Read the model definition and answer for the solid it produces. Units are mm, in the model's axes. Coordinates: 2 decimals unless noted, no trailing zeros. Write each loop counter-clockwise with the first axis right and the second up, starting at its lowest first coordinate (ties: lowest second). Pieces come first, ordered by that corner, then holes.
Item 1: Section B-B (z = 0) is taken. Give the vertices of the cut face in (x, y), then the cut area to 3 significant figures.
Item 2: Section D-D (y = 9) is taken. Give the vertices of the cut face in (x, z).
Item 3: Section C-C (y = 0) is taken. Give the vertices of the cut face in (x, z).
Item 4: Section A-A (x = 0) is taken. Give the vertices of the cut face in (y, z).
Item 5: Each of these flat-tipped pins is pushed along its axis until it touches: P1, Ø5, axis at y = -30, z = -0.5, coming from the -X side; P2, Ø5, axis at x = -25, y = -25.5, coming from the +Z side; P3, Ø3, axis at y = -15.5, z = 20.5, coming from the -X side. Where does it stop, or does it pass through?
Item 6: Determine the mould class of faces 1 (the face through (1, 40, -1)), 2 (the face through (1, -40, -1)), 3 (the face through (13.41, 32.33, 0.55)) for opening direction Y: released by +Y, released by -Y, zero draft, split by the parting line, or undercut.
Item 7: Straight lines are drawn through the part: probe 1 along Y at (x, z) = (0, -4); probe 2 along X at (y, z) = (0, -1); probe 3 along X at (y, z) = (0, -14.5). For each, find the intervals that lie inside material, in ascending order.
from build123d import *

# Parameters (mm, degrees)
SCHIZZO1_R        = 39
ESTRUSIONE1_DEPTH = 40
SCHIZZO3_R        = 35
ESTRUSIONE3_DEPTH = 40
SMUSSO1_SIZE      = 1


with BuildPart() as part:
    # Schizzo1 → Estrusione1 (new, symmetric)
    with BuildSketch(Plane(origin=(0, 0, 0), x_dir=(1, 0, 0), z_dir=(0, 1, 0))):
        with Locations(Location((0, 0, 0), (0, 0, 270))):
            Circle(SCHIZZO1_R)
    extrude(amount=ESTRUSIONE1_DEPTH, both=True)

    # Schizzo3 → Estrusione3 (cut, symmetric)
    with BuildSketch(Plane.XY):
        with Locations(Location((0, 0, 0), (0, 0, 90))):
            Circle(SCHIZZO3_R)
    extrude(amount=ESTRUSIONE3_DEPTH, both=True, mode=Mode.SUBTRACT)

    # Smusso1
    smusso1_edges = [part.edges().sort_by_distance(p)[0] for p in [
        (0, 40, -39),
    ]]
    chamfer(smusso1_edges, length=SMUSSO1_SIZE)


solid = part.part
Established:
1. outline: (-39, -40) - (39, -40) - (39, 39) - (38, 40) - (-38, 40) - (-39, 39) - close; hole circle Ø70 at (0, 0)
1. area: 2,390 mm2
2. outline: (-33.82, -19.42) - (-33.82, 19.42) arc R39 ccw to start; (33.82, -19.42) arc R39 ccw to (33.82, 19.42) - close
3. outline: (-35, -17.2) - (-35, 17.2) arc R39 ccw to start; (35, -17.2) arc R39 ccw to (35, 17.2) - close
4. outline: (-40, -39) - (-35, -39) - (-35, 39) - (-40, 39) - close; (35, -39) - (39, -39) - (40, -38) - (40, 38) - (39, 39) - (35, 39) - close
5. P1: stops at x = -39
5. P2: stops at z = 31.68
5. P3: stops at x = -34.06
6. face 1: released by +Y
6. face 2: released by -Y
6. face 3: undercut
7. probe 1: y = -40 to -35, 35 to 40
7. probe 2: x = -38.99 to -35, 35 to 38.99
7. probe 3: x = -36.2 to -35, 35 to 36.2
